from build123d import *

# Parameters (mm, degrees)
SKETCH1_R           = 25
SKETCH1_R_2         = 3
SKETCH1_R_3         = 1.25
BOSS_EXTRUDE1_DEPTH = 15
SKETCH2_R           = 20
CUT_EXTRUDE1_DEPTH  = 11
FILLET1_R           = 2
BOSS_EXTRUDE2_DEPTH = 15
CIRPATTERN1_COUNT   = 20


with BuildPart() as part:
    # Sketch1 → Boss-Extrude1 (new body)
    with BuildSketch(Plane(origin=(0, 0, 0), x_dir=(1, 0, 0), z_dir=(0, 1, 0))):
        with Locations(Location((0, 0, 0), (0, 0, 270))):
            Circle(SKETCH1_R)
        with Locations(Location((0, 0, 0), (0, 0, 270))):
            Circle(SKETCH1_R_2, mode=Mode.SUBTRACT)
        with Locations(Location((0, 8, 0), (0, 0, 270))):
            Circle(SKETCH1_R_3, mode=Mode.SUBTRACT)
        with Locations(Location((8, 0, 0), (0, 0, 270))):
            Circle(SKETCH1_R_3, mode=Mode.SUBTRACT)
        with Locations(Location((0, -8, 0), (0, 0, 270))):
            Circle(SKETCH1_R_3, mode=Mode.SUBTRACT)
        with Locations(Location((-8, 0, 0), (0, 0, 270))):
            Circle(SKETCH1_R_3, mode=Mode.SUBTRACT)
    extrude(amount=BOSS_EXTRUDE1_DEPTH)

    # Sketch2 → Cut-Extrude1 (cut)
    with BuildSketch(Plane(origin=(0, 15, 0), x_dir=(1, 0, 0), z_dir=(0, 1, 0))):
        with Locations(Location((0, 0, 0), (0, 0, 270))):
            Circle(SKETCH2_R)
    extrude(amount=-CUT_EXTRUDE1_DEPTH, mode=Mode.SUBTRACT)

    # Fillet1
    fillet1_edges = [part.edges().sort_by_distance(p)[0] for p in [
        (0, 4, -20),
        (0, 15, -20),
    ]]
    fillet(fillet1_edges, radius=FILLET1_R)

    # Sketch3 → Boss-Extrude2 (add)
    with BuildSketch(Plane.XZ):
        with BuildLine():
            Line((1.175860097, -24.094064846), (1.034143555, -26.297367496))
            ThreePointArc((1.034143555, -26.297367496), (0.877193006, -26.629997556), (0.535174624, -26.765273788))
            Line((0.535174624, -26.765273788), (-0.535174624, -26.765273788))
            ThreePointArc((-0.535174624, -26.765273788), (-0.877193006, -26.629997556), (-1.034143555, -26.297367496))
            Line((-1.034143555, -26.297367496), (-1.175860097, -24.094064846))
            Line((-1.175860097, -24.094064846), (1.175860097, -24.094064846))
        make_face()
    boss_extrude2 = extrude(amount=-BOSS_EXTRUDE2_DEPTH)

    # CirPattern1: Boss-Extrude2 ×20 about axis
    cirpattern1_axis = Axis((0, 0, 0), (0, 1, 0))
    for i in range(1, CIRPATTERN1_COUNT):
        add(boss_extrude2.rotate(cirpattern1_axis, i * 360 / CIRPATTERN1_COUNT))


solid = part.part
Part model, mm, in its own coordinate system. A direction names the side the tool comes from. Round coordinates to 2 decimals unless told otherwise and drop trailing zeros. Answer as a JSON object with one key per item and string values.
Item 1: Tool access for faces 5 (the face through (17.65, 7.395, 17.705)), 6 (the face through (-25.645, 7.395, 1.076)), 7 (the face through (24.72, 7.4, 6.9)), 8 (the face through (-3.87, 7.4, -24.7)), 9 (the face through (-1.077, 7.395, 25.627)): list every direction of +Z, -Z, +X, -X, +Y, -Y with a clear straight run to the whole face (end or side of a thin tool).
Output:
{"face 5": "+Y, -Y", "face 6": "-X, +Y, -Y", "face 7": "+X, +Y, -Y", "face 8": "-Z, +Y, -Y", "face 9": "+Z, +Y, -Y"}
Item 2: Pull direction X, two halves, no side cores. Call faces 1 (the face through (25.627, 7.395, 1.077)), 2 (the face through (-4, 15, -22)), 3 (the face through (-24.686, 7.395, -3.95)), 4 (the face through (-17.65, 7.395, -17.705)): pulls with the +X half, pulls with the -X half, needs draft (parallel to the pull), parting line crosses it, or undercut.
Output:
{"face 1": "pulls with the +X half", "face 2": "needs draft", "face 3": "pulls with the -X half", "face 4": "undercut"}
Item 3: Wall check: L1, parallel to X at y = 0.8, z = 0; L2, parallel to Z at x = 0.5, y = 6.75. Give the ranges that are in metal, low to high.
Output:
{"L1": "-26.77 to -9.25, -6.75 to -3, 3 to 6.75, 9.25 to 26.77", "L2": "-26.77 to -19.99, 19.99 to 26.77"}
Item 4: Pin check, flat tips, straight feed: pin 1 (10 mm diameter, centred on x = 20.5, z = -19, fed in from -Y); pin 2 (1.5 mm diameter, centred on x = -18.5, y = 12, fed in from -Z); pin 3 (4 mm diameter, centred on x = -8, z = 0, fed in from +Y); pin 4 (1 mm diameter, centred on y = 6, z = -12, fed in from +X). Stop position of each tip, or through.
Output:
{"pin 1": "y = 0", "pin 2": "z = -17.61", "pin 3": "y = 4", "pin 4": "x = 22.2"}
Item 5: Band-saw the part on A-A on y = 2.5. State how many separate pieces and enclosed holes the cut face has, plus the area to 3 significant figures.
Output:
{"separate pieces": "1", "enclosed holes": "5", "area": "1,990 mm2"}
